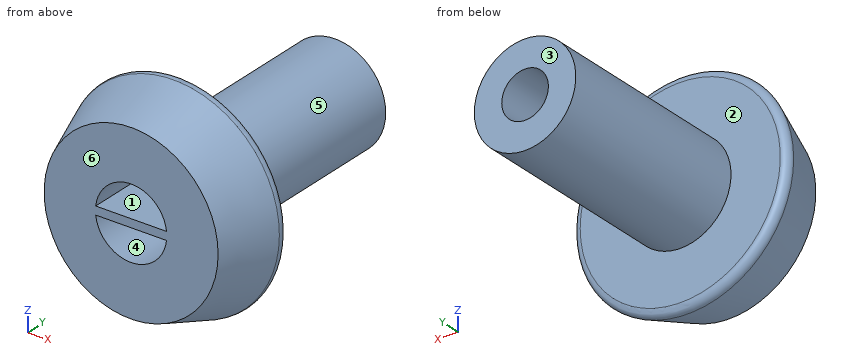
from build123d import *

# Parameters (mm, degrees)
F3_DEPTH = 7.62
F4_R     = 0.635


with BuildPart() as f1:
    # F0 (on Top) → F1 (revolve)
    with BuildSketch(Plane.XY):
        Polygon((3.302, 7.62), (3.302, 4.826), (8.0532941176, 4.826), (10.16, 10.795), (4.699, 10.795), (3.302, 10.795), align=None)
        Polygon((0, 17.145), (0, 12.446), (3.302, 12.446), (3.302, 10.795), (4.699, 10.795), (4.699, 29.845), (2.159, 29.845), (2.159, 17.145), align=None)
    revolve(axis=Axis((0, 23.495, 0), (0, 1, 0)))

    # F2 (on face) → F3 (join)
    with BuildSketch(Plane.XZ.offset(-12.446)):
        with BuildLine():
            ThreePointArc((-3.2799455788, 0.381), (-3.302, 0), (-3.2799455788, -0.381))
            Line((-3.2799455788, -0.381), (3.2799455788, -0.381))
            ThreePointArc((3.2799455788, -0.381), (3.2964817838, -0.1908188916), (3.302, 0))
            ThreePointArc((3.302, 0), (3.2964817838, 0.1908188916), (3.2799455788, 0.381))
            Line((3.2799455788, 0.381), (-3.2799455788, 0.381))
        make_face()
    extrude(amount=F3_DEPTH)

    # F4
    f4_edges = [f1.edges().sort_by_distance(p)[0] for p in [
        (-10.16, 10.795, 0),
    ]]
    fillet(f4_edges, radius=F4_R)


solid = f1.part
Input: part model. Units: mm. Frame: model coordinates. Face numbers are marked on the shaded views. A direction names the side the tool comes from. Round coordinates to 2 decimals unless told otherwise and drop trailing zeros. Write each loop counter-clockwise with the first axis right and the second up, starting at its lowest first coordinate (ties: lowest second). Pieces come first, ordered by that corner, then holes.
1) Ray query, L1, parallel to X at y = 22, z = 0; L2, parallel to X at y = 19.5, z = -1. Return the intervals inside material, ascending.
2) Cut plane C-C (y = 25.5). Return the cut outline in (x, z), then the cut area to 3 significant figures.
3) Contact query for flat-ended pins moving along their axis: P1, Ø1.5, axis at y = 15.5, z = -3, coming from the -X side; P2, Ø2, axis at y = 8, z = -2, coming from the -X side; P3, Ø4, axis at x = 0, z = 0, coming from the +Y side (3 decimals). Output: stop coordinate, or through.
4) Cut plane B-B (x = 0). Return the cut outline in (y, z) (1 decimal).
5) Draft query along X for the marked faces 4, 5 and 6. Return one class per face: pulls with the +X half, pulls with the -X half, needs draft (parallel to the pull), parting line crosses it, or undercut.
6) Reachability of the marked faces 1, 2 and 3 from +Z, -Z, +X, -X, +Y, -Y: full face, straight path, thin tool, end or side. Return the list, or none.
7) Cut plane A-A (z = 0). Return the cut outline in (x, y) (1 decimal), then the cut area to 3 significant figures.
Geometry says:
1. L1: x = -4.7 to -2.16, 2.16 to 4.7
1. L2: x = -4.59 to -1.91, 1.91 to 4.59
2. outline: circle Ø9.4 at (0, 0); hole circle Ø4.32 at (0, 0)
2. area: 54.7 mm2
3. P1: stops at x = -4.13
3. P2: stops at x = -9.36
3. P3: stops at y = 17.145
4. outline: (4.8, -8.1) - (9.9, -9.9) arc R0.6 ccw to (10.8, -9.3) - (10.8, -4.7) - (29.8, -4.7) - (29.8, -2.2) - (17.1, -2.2) - (17.1, 2.2) - (29.8, 2.2) - (29.8, 4.7) - (10.8, 4.7) - (10.8, 9.3) arc R0.6 ccw to (9.9, 9.9) - (4.8, 8.1) - (4.8, 3.3) - (12.4, 3.3) - (12.4, 0.4) - (4.8, 0.4) - (4.8, -0.4) - (12.4, -0.4) - (12.4, -3.3) - (4.8, -3.3) - close
5. face 4: undercut
5. face 5: parting line crosses it
5. face 6: needs draft
6. face 1: -Y
6. face 2: +Y
6. face 3: +Z, -Z, +X, -X, +Y
7. outline: (-9.9, 9.9) - (-8.1, 4.8) - (8.1, 4.8) - (9.9, 9.9) arc R0.6 ccw to (9.3, 10.8) - (4.7, 10.8) - (4.7, 29.8) - (2.2, 29.8) - (2.2, 17.1) - (-2.2, 17.1) - (-2.2, 29.8) - (-4.7, 29.8) - (-4.7, 10.8) - (-9.3, 10.8) arc R0.6 ccw to start
7. area: 233 mm2
